Here's the drawing with two shaded views (mm, measured from the low corner). I have some questions. A direction names the side the tool comes from. Give positions to 0.01 mm unless a question says otherwise; leave off trailing zeros. Loops run counter-clockwise (first coordinate to the right, second up) from the corner with the lowest first, then second, coordinate; pieces in that order, holes last.
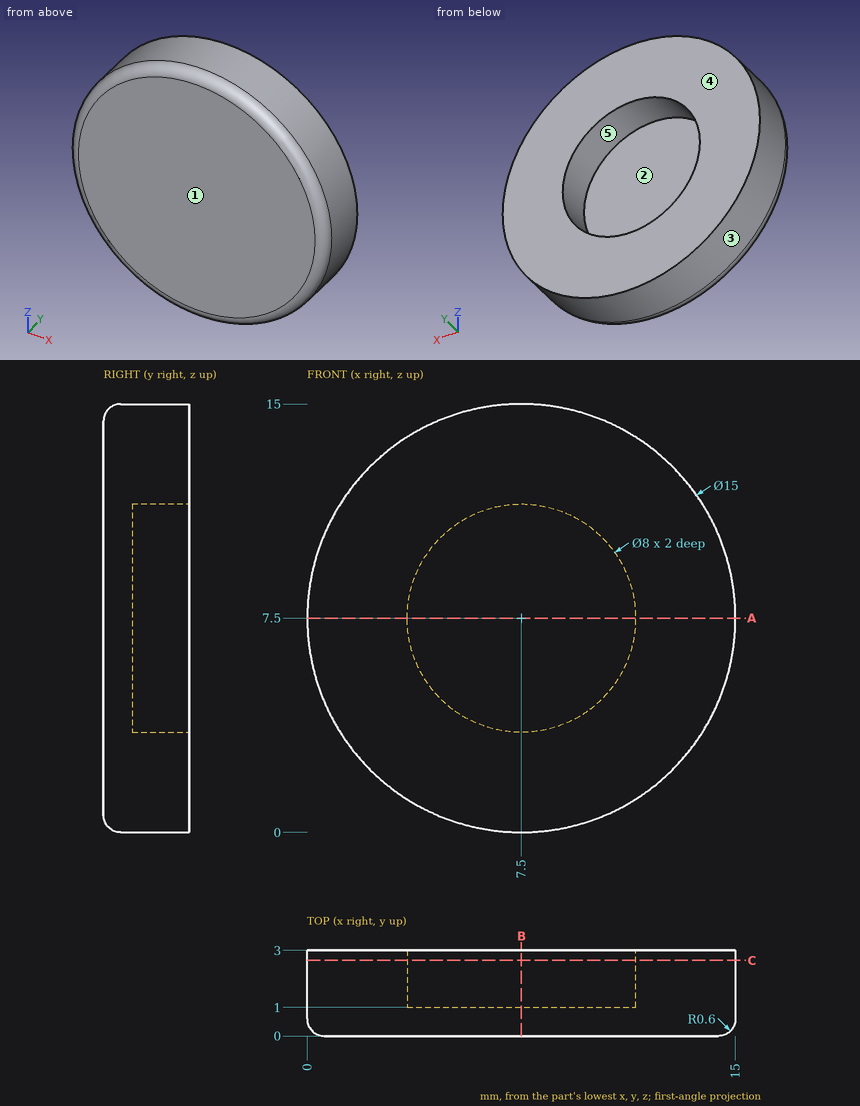
(1) Please list where these lines run through material, in increasing order: probe 1 along Z at (x, y) = (7.5, 1.6); probe 2 along Y at (x, z) = (9.5, 9.75); probe 3 along Z at (x, y) = (4.25, 2.3).
Returned:
probe 1: z = 0 to 3.5, 11.5 to 15
probe 2: y = 0 to 1
probe 3: z = 0.74 to 5.17, 9.83 to 14.26
(2) Suppose I cut it at B-B on x = 7.5. List the corners of the cut face in (y, z) for me, plus the area to 3 significant figures.
Returned:
outline: (0, 0.6) arc R0.6 ccw to (0.6, 0) - (3, 0) - (3, 3.5) - (1, 3.5) - (1, 11.5) - (3, 11.5) - (3, 15) - (0.6, 15) arc R0.6 ccw to (0, 14.4) - close
area: 28.8 mm2
(3) Suppose I cut it at C-C on y = 2.65. List the corners of the cut face in (x, z) for me.
Returned:
outline: circle Ø15 at (7.5, 7.5); hole circle Ø8 at (7.5, 7.5)
(4) Will these pins go through, and if not, where does the flat tip stop? P1, Ø8, axis at x = 11, z = 9, coming from the +Y side; P2, Ø4, axis at x = 6.5, z = 7.5, coming from the +Y side; P3, Ø1, axis at y = 2.5, z = 12, coming from the -X side; P4, Ø1, axis at x = 13, z = 1.5, coming from the +Y side.
Returned:
P1: stops at y = 3
P2: stops at y = 1
P3: stops at x = 1.16
P4: passes through
(5) Thinking about a two-plate mould opening in X: for the marked faces 1, 2 and 3, which applies, pulls with the +X half, pulls with the -X half, needs draft (parallel to the pull), parting line crosses it, or undercut?
Returned:
face 1: needs draft
face 2: undercut
face 3: parting line crosses it
(6) Suppose I cut it at A-A on z = 7.5. List the corners of the cut face in (x, y) for me, plus the area to 3 significant figures.
Returned:
outline: (0, 0.6) arc R0.6 ccw to (0.6, 0) - (14.4, 0) arc R0.6 ccw to (15, 0.6) - (15, 3) - (11.5, 3) - (11.5, 1) - (3.5, 1) - (3.5, 3) - (0, 3) - close
area: 28.8 mm2
(7) Which directions (+Z, -Z, +X, -X, +Y, -Y) give clear straight access to the entire face, cutting with the end or side of a thin tool? Please do the marked faces 4 and 5.
Returned:
face 4: +Z, -Z, +X, -X, +Y
face 5: +Y
